Autodesk Inventor part; units mm, degrees
ref_plane "YZ Plane" through (0, 0, 0) normal (1, 0, 0) x (0, 1, 0)
ref_plane "XZ Plane" through (0, 0, 0) normal (0, 1, 0) x (-1, 0, 0)
ref_plane "XY Plane" through (0, 0, 0) normal (0, 0, 1) x (1, 0, 0)
sketch "Sketch1" plane through (0, 0, 0) normal (0, 1, 0) x (-1, 0, 0)
  line L0 (-20, -115) -> (20, -115)
  line L1 (25, -110) -> (25, 110)
  line L2 (20, 115) -> (-20, 115)
  line L3 (-25, 110) -> (-25, -110)
  line L4 (-5, -105) -> (5, -105)
  line L5 (5, -105) -> (5, 105)
  line L6 (5, 105) -> (-5, 105)
  line L7 (-5, 105) -> (-5, -105)
  arc A0 (25, 110) -> (20, 115) centre (20, 110) ccw
  arc A1 (-20, 115) -> (-25, 110) centre (-20, 110) ccw
  arc A2 (-25, -110) -> (-20, -115) centre (-20, -110) ccw
  arc A3 (20, -115) -> (25, -110) centre (20, -110) ccw
  line L8 (-1.5, -105) -> (1.5, -105)
  line L9 (1.5, 105) -> (-1.5, 105)
  point P0 (0, 0)
  point P1 (0, 0)
  dimension "d6" = 10
  dimension "d7" = 210
  dimension "d8" = 5
  dimension "d9" = 3
  dimension "d10" = 210
extrude "Extrusion1" add sketch "Sketch1" along normal blind 30
extrude "Extrusion2" add sketch "Sketch1" along normal blind 15 contours L7 L6 L5 L4
sketch "Sketch2" plane through (0, 30, 0) normal (0, 1, 0) x (1, 0, 0)
  line L0 (-1.5, -105) -> (1.5, -105)
  line L1 (1.5, -105) -> (1.5, 105)
  line L2 (1.5, 105) -> (-1.5, 105)
  line L3 (-1.5, 105) -> (-1.5, -105)
  line L4 (-1.5, -105) -> (1.5, 105) construction
  line L5 (1.5, -105) -> (-1.5, 105) construction
  line L6 (5, 105) -> (5, -105)
  line L7 (5, 105) -> (1.5, 105)
  line L8 (1.5, 105) -> (1.5, -105)
  line L9 (1.5, -105) -> (5, -105)
  line L10 (5, -105) -> (5, 105)
  line L11 (-5, 105) -> (5, 105)
  line L12 (-5, 105) -> (-1.5, 105)
  line L13 (-1.5, 105) -> (-1.5, -105)
  line L14 (-1.5, -105) -> (-5, -105)
  line L15 (-5, -105) -> (-5, 105)
  point P0 (0, 0)
  dimension "d15" = 3
  dimension "d16" = 210
extrude "Extrusion3" add sketch "Sketch2" against normal blind 15 contours L14 L15 L11 L3 | L1 L7 L6 L9
sketch "Sketch5" plane through (-20, 0, 115) normal (0, 0, 1) x (1, 0, 0)
  line L0 (15.5, 15) -> (24.5, 15)
  line L1 (25.5, 16) -> (25.5, 17.5)
  line L2 (24.5, 18.5) -> (15.5, 18.5)
  line L3 (14.5, 17.5) -> (14.5, 16)
  arc A0 (15.5, 18.5) -> (14.5, 17.5) centre (15.5, 17.5) ccw
  arc A1 (14.5, 16) -> (15.5, 15) centre (15.5, 16) ccw
  arc A2 (24.5, 15) -> (25.5, 16) centre (24.5, 16) ccw
  arc A3 (25.5, 17.5) -> (24.5, 18.5) centre (24.5, 17.5) ccw
  line L4 (-5, 0) -> (-5, 30)
  point P0 (20, 0)
  point P1 (14.5, 15)
  point P2 (25.5, 18.5)
  point P3 (25.5, 15)
  point P4 (14.5, 18.5)
  point P5 (14.5, 16.75)
  dimension "d23" = 11
  dimension "d24" = 3.5
  dimension "d27" = 1
  dimension "d38" = 19.5
extrude "Extrusion4" cut sketch "Sketch5" against normal blind 225
ref_plane "Work Plane1" through (0, 18.5, 0) normal (0, 1, 0) x (1, 0, 0)
sketch "Sketch6" plane through (0, 18.5, 0) normal (0, 1, 0) x (1, 0, 0)
  line L0 (-1.5, -105) -> (1.5, -105)
  line L1 (1.5, -105) -> (1.5, -101.5)
  line L2 (1.5, -101.5) -> (-1.5, -101.5)
  line L3 (-1.5, -101.5) -> (-1.5, -105)
  line L4 (0, 0) -> (38.1374, 0)
  line L5 (-1.5, 105) -> (1.5, 105)
  line L6 (1.5, 105) -> (1.5, 101.5)
  line L7 (1.5, 101.5) -> (-1.5, 101.5)
  line L8 (-1.5, 101.5) -> (-1.5, 105)
  dimension "d31" = 3.5
extrude "Extrusion5" add sketch "Sketch6" along normal blind 4.5
ref_plane "Work Plane2" through (0, 12.5, 0) normal (0, 1, 0) x (1, 0, 0)
move faces "Move1" translate (0, 12, 0) faces at (8.3333, 0, 36.6667)
properties part number "acrylic_base"
Part model, mm, in its own coordinate system. A direction names the side the tool comes from. Round coordinates to 2 decimals unless told otherwise and drop trailing zeros. Loops run counter-clockwise (first coordinate to the right, second up) from the corner with the lowest first, then second, coordinate; pieces in that order, holes last.
1. Two-plate mould, pull along Z, no slides. Class faces 1 (the face through (0, 21, -115)), 2 (the face through (0, 21, 115)), 3 (the face through (0, 12, 2)), 4 (the face through (1.5, 24, 1)): pulls with the +Z half, pulls with the -Z half, needs draft (parallel to the pull), parting line crosses it, or undercut.
Solutions:
face 1: pulls with the -Z half
face 2: pulls with the +Z half
face 3: needs draft
face 4: undercut
2. 3-axis set-ups, long thin cutter, end or side, ignore diameter. For faces 5 (the face through (-24, 21, -113)), 6 (the face through (-1.5, 24, -1)), 7 (the face through (2, 18.5, 4)): which of +Z, -Z, +X, -X, +Y, -Y reach the whole face in a straight line?
Solutions:
face 5: -Z, -X, +Y, -Y
face 6: +Y
face 7: +Z
3. Slice it at B-B (z = -56.5). Give the cut face in (x, y).
Solutions:
outline: (-25, 12) - (25, 12) - (25, 30) - (1.5, 30) - (1.5, 18.5) - (4.5, 18.5) arc R1 cw to (5.5, 17.5) - (5.5, 16) arc R1 cw to (4.5, 15) - (-4.5, 15) arc R1 cw to (-5.5, 16) - (-5.5, 17.5) arc R1 cw to (-4.5, 18.5) - (-1.5, 18.5) - (-1.5, 30) - (-25, 30) - close
4. Slice it at A-A (y = 21). Give the cut face in (x, z).
Solutions:
outline: (-25, -110) arc R5 ccw to (-20, -115) - (20, -115) arc R5 ccw to (25, -110) - (25, 110) arc R5 ccw to (20, 115) - (-20, 115) arc R5 ccw to (-25, 110) - close; hole (-1.5, -101.5) - (1.5, -101.5) - (1.5, 101.5) - (-1.5, 101.5) - close
5. Drill centre lines: line 1 along Y through (x, z) = (4, -48); line 2 along X through (y, z) = (17.5, 64); line 3 along X through (y, z) = (27.5, -75). Where is each one in solid material? Low to high.
Solutions:
line 1: y = 12 to 15, 18.5 to 30
line 2: x = -25 to -5.5, 5.5 to 25
line 3: x = -25 to -1.5, 1.5 to 25
6. Flat gauge pin, fed straight in: pin 1 (0.9 mm diameter, centred on x = -0.5, z = 104, fed in from +Y). Where does the tip first touch, or does it go through?
Solutions:
pin 1: stops at y = 23
